Source: CAD feature listing. Evaluate the final solid. Frame: model axes, mm. Face numbers are marked on the shaded views. A direction names the side the tool comes from. Give positions to 0.01 mm unless a question says otherwise; leave off trailing zeros. Order: outer loops, then holes, each group sorted by start corner. A loop starts at its lowest first (then second) coordinate and runs counter-clockwise, first axis right, second up.
1) Material intervals for line 1 (Y direction, x = -0.5, z = 5.45); line 2 (Y direction, x = 0, z = 3); line 3 (X direction, y = 19, z = 3.05), sorted ascending.
2) Section A-A, the plane z = 5.1. Return loops of the section in (x, y).
3) Section C-C, the plane y = 10. Return loops of the section in (x, z).
4) Section B-B, the plane x = 0. Return loops of the section in (y, z), plus the area to 3 significant figures.
5) Section D-D, the plane x = 13.5. Return loops of the section in (y, z).
6) Draft query along Y for the marked faces 3, 4 and 5. Return one class per face: released by +Y, released by -Y, zero draft, split by the parting line, or undercut.
7) Access query for the marked faces 1 and 2. Directions: +Z, -Z, +X, -X, +Y, -Y. A direction counts if a zero-diameter tool reaches every point of the face in a straight line with its end or side. Return the directions, or none.
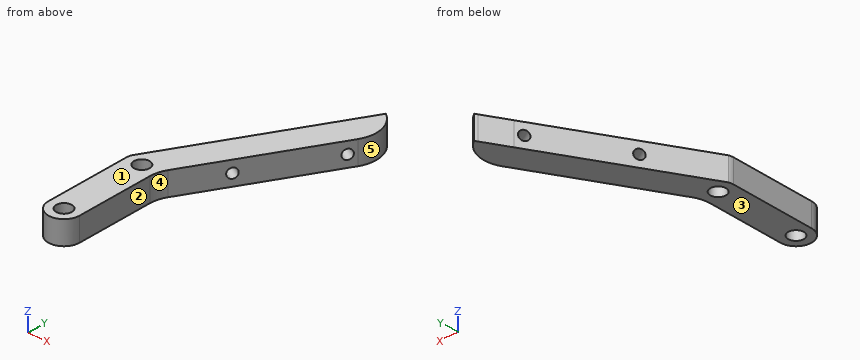
Autodesk Inventor part; units mm, degrees
ref_plane "YZ Plane" through (0, 0, 0) normal (1, 0, 0) x (0, 1, 0)
ref_plane "XZ Plane" through (0, 0, 0) normal (0, 1, 0) x (-1, 0, 0)
ref_plane "XY Plane" through (0, 0, 0) normal (0, 0, 1) x (1, 0, 0)
sketch "Sketch1" plane through (0, 0, 0) normal (0, 0, 1) x (1, 0, 0)
  circle A0 centre (0, 0) radius 2
  arc A1 (-4, 0) -> (4, 0) centre (0, 0) ccw
  line L0 (0, 0) -> (0, 22) construction
  circle A2 centre (0, 22) radius 2
  arc A3 (-3.7993, 23.2511) -> (-4, 22) centre (0, 22) ccw
  line L1 (0, 22) -> (25, 65.3013) construction
  circle A4 centre (25, 65.3013) radius 2
  arc A5 (27, 61.8372) -> (21.2007, 66.5524) centre (25, 65.3013) ccw
  line L2 (-4, 0) -> (-4, 22)
  line L3 (4, 0) -> (4, 22)
  line L4 (-3.7993, 23.2511) -> (17.6088, 60.331)
  line L5 (24, 56.641) -> (4, 22)
  line L6 (30.6468, 62.0411) -> (28.537, 63.2592)
  line L7 (27, 61.8372) -> (28, 63.5692)
  line L8 (21.2007, 66.5524) -> (17.6088, 60.331)
  line L9 (21.0718, 67.5692) -> (19.4047, 68.5317)
  line L10 (21.2007, 66.5524) -> (21.6088, 67.2592)
  arc A6 (24, 56.641) -> (21.0718, 67.5692) centre (17.0718, 60.641) ccw
  line L11 (27, 61.8372) -> (24, 56.641)
  point P0 (21.5269, 67.2857)
  point P1 (21.5967, 67.2384)
  dimension "d0" = 4
  dimension "d1" = 8
  dimension "d2" = 22
  dimension "d3" = 4
  dimension "d4" = 8
  dimension "d5" = 50
  dimension "d6" = 150
  dimension "d7" = 4
  dimension "d8" = 8
  dimension "d13" = 8
extrude "Extrusion1" add sketch "Sketch1" along normal blind 6 contours L2 A3 L4 L8 L10 A6 A4 L5 L3 A1 | A4 A6 picked at (23.7732, 64.4877)
fillet "Fillet1" radius 8 1 edges at (4, 22, 3)
sketch "Sketch2" plane through (-3.7993, 23.2511, 0) normal (-0.866, 0.5, 0) x (0, 0, 1)
  line L0 (0, 42.8162) -> (6, 42.8162)
  circle A0 centre (3, 17.7921) radius 1.25
  circle A1 centre (3, 40.7921) radius 1.25
  line L1 (0, 50.7921) -> (6, 50.7921)
  line L2 (0, 0) -> (6, 0)
  line L3 (-2.4062, 7.7921) -> (9.3174, 7.7921)
  point P0 (0, -18.2364)
  dimension "d15" = 2.5
  dimension "d16" = 2.5
  dimension "d17" = 10
  dimension "d19" = 43
  dimension "d20" = 10
extrude "Extrusion2" cut sketch "Sketch2" against normal blind 10
properties part number "Gripper 5-2"
From the geometry:
1. line 1: y = -3.97 to -1.94, 1.94 to 20.06, 23.94 to 28.97
1. line 2: y = -4 to -2, 2 to 20, 24 to 29.83
1. line 3: x = -4 to 4
2. outline: (-4, 0) arc R4 ccw to (4, 0) - (4, 19.86) arc R8 cw to (5.07, 23.86) - (24, 56.64) arc R8 ccw to (21.6, 67.24) - (21.2, 66.55) - (17.61, 60.33) - (-3.8, 23.25) arc R4 ccw to (-4, 22) - close; hole circle Ø4 at (0, 0); hole circle Ø4 at (0, 22)
3. outline: (-4, 0) - (4, 0) - (4, 6) - (-4, 6) - close
4. outline: (-4, 0) - (-2, 0) - (-2, 6) - (-4, 6) - close; (2, 0) - (20, 0) - (20, 6) - (2, 6) - close; (24, 0) - (29.83, 0) - (29.83, 6) - (24, 6) - close
4. area: 155 mm2
5. outline: (38.45, 0) - (53.21, 0) - (53.21, 6) - (38.45, 6) - close
6. face 3: zero draft
6. face 4: released by -Y
6. face 5: split by the parting line
7. face 1: +Z, +X, -X, +Y, -Y
7. face 2: +Z, -Z, +X, -Y
